Source: three-view drawing plus pictorial views. Frame: mm from the lowest corner of the part. Give positions to 0.01 mm unless a question says otherwise; leave off trailing zeros. Write each loop counter-clockwise with the first axis right and the second up, starting at its lowest first coordinate (ties: lowest second). Pieces come first, ordered by that corner, then holes. Notation, with made-up numbers: (21.25, 49) -> (72.25, 49) arc R19 cw to (72.25, 74) -> close; hole circle Ø7 at (80.5, 58). An arc over 180 degrees is marked (long way). Write item = value, one per line.
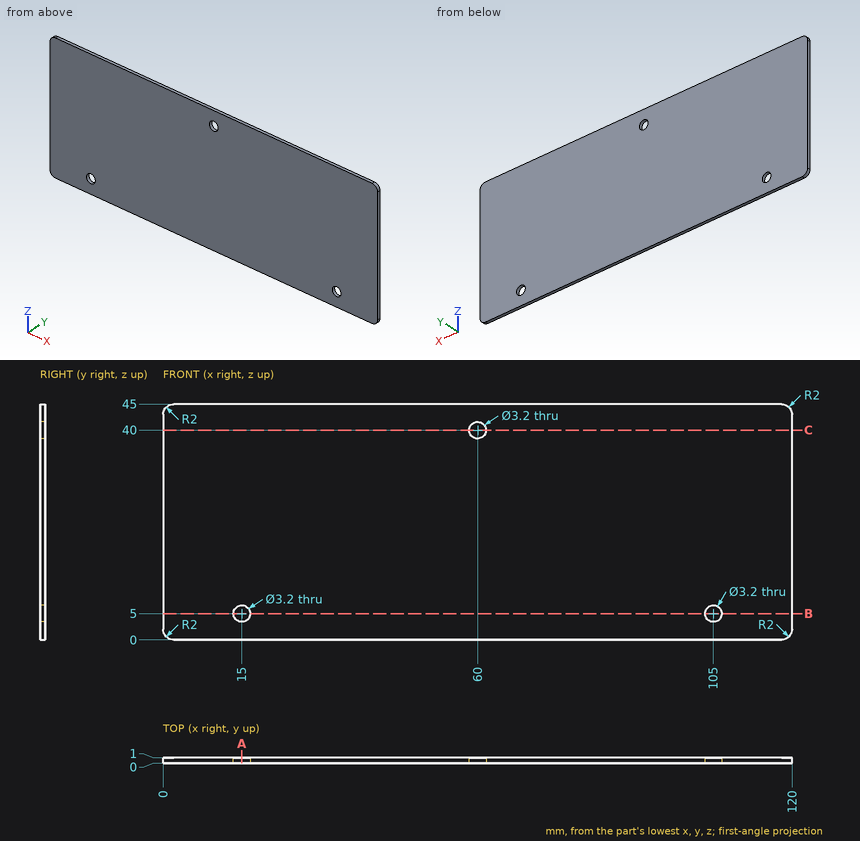
1) Cut plane A-A (x = 15). Return the cut outline in (y, z).
Computed:
outline = (0, 0) -> (1, 0) -> (1, 3.4) -> (0, 3.4) -> close; (0, 6.6) -> (1, 6.6) -> (1, 45) -> (0, 45) -> close
2) Contact query for a flat-ended pin moving along its axis: pin 1 (2.5 mm diameter, centred on x = 15, z = 5, fed in from -Y). Output: stop coordinate, or through.
Computed:
pin_1 = through
3) Cut plane B-B (z = 5). Return the cut outline in (x, y), then the cut area to 3 significant figures.
Computed:
outline = (0, 0) -> (13.4, 0) -> (13.4, 1) -> (0, 1) -> close; (16.6, 0) -> (103.4, 0) -> (103.4, 1) -> (16.6, 1) -> close; (106.6, 0) -> (120, 0) -> (120, 1) -> (106.6, 1) -> close
area = 114 mm²
4) Material intervals for L1, parallel to Z at x = 105, y = 0.3; L2, parallel to Z at x = 60, y = 0.5; L3, parallel to X at y = 0.2, z = 41, sorted ascending.
Computed:
L1 = 0 to 3.4, 6.6 to 45
L2 = 0 to 38.4, 41.6 to 45
L3 = 0 to 58.75, 61.25 to 120
5) Cut plane C-C (z = 40). Return the cut outline in (x, y).
Computed:
outline = (0, 0) -> (58.4, 0) -> (58.4, 1) -> (0, 1) -> close; (61.6, 0) -> (120, 0) -> (120, 1) -> (61.6, 1) -> close
